Here's the drawing with two shaded views (mm, measured from the low corner). I have some questions. Coordinates: 2 decimals unless noted, no trailing zeros. Loops run counter-clockwise (first coordinate to the right, second up) from the corner with the lowest first, then second, coordinate; pieces in that order, holes last.
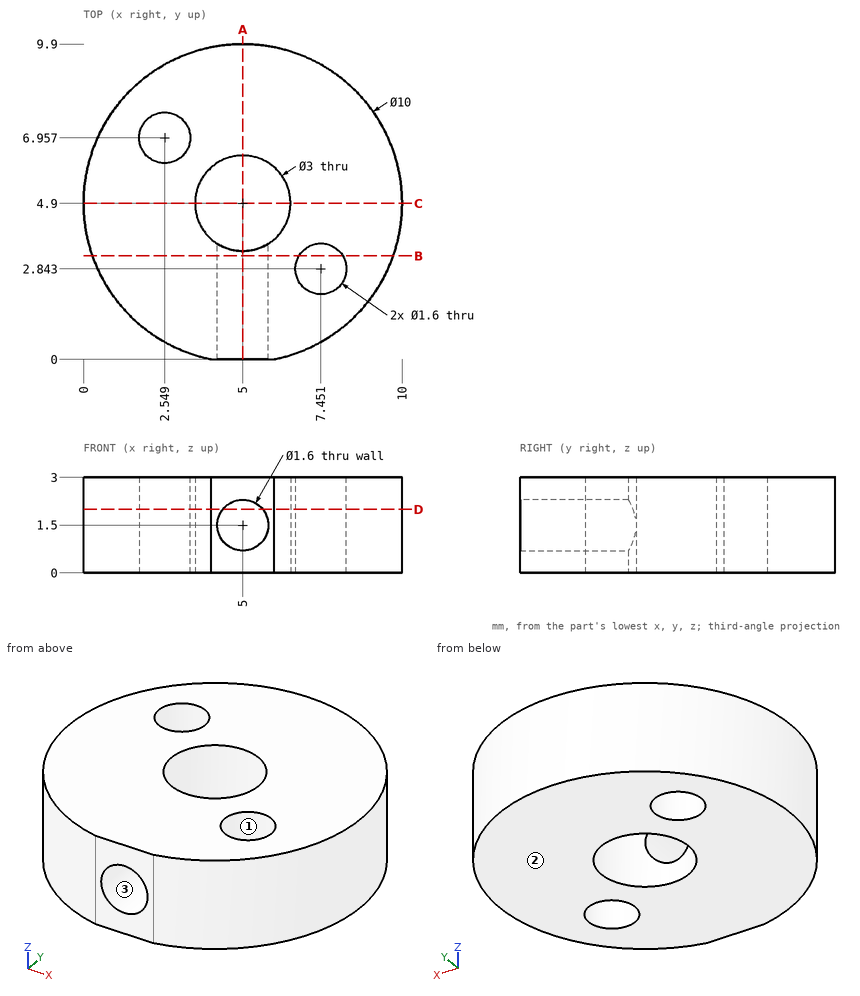
Q1. Suppose I cut it at D-D on z = 2. State how many separate pieces and enclosed holes the cut face has.
Q2. We'd pull the mould along Z, two halves only. Please class the marked faces 1, 2 and 3: pulls with the +Z half, pulls with the -Z half, needs draft (parallel to the pull), parting line crosses it, or undercut.
Q3. Suppose I cut it at A-A on x = 5. Write out the boundary of the cut face in (y, z).
Q4. Suppose I cut it at C-C on y = 4.9. Write out the boundary of the cut face in (x, z).
Q5. Will these pins go through, and if not, where does the flat tip stop? P1, Ø1.5, axis at x = 3.5, z = 1, coming from the +Y side; P2, Ø1.3, axis at x = 7.45, y = 2.84, coming from the +Z side.
Q6. Please list where these lines run through material, in increasing order: probe 1 along X at (y, z) = (1.35, 1.5); probe 2 along X at (y, z) = (1.8, 1.5); probe 3 along Y at (x, z) = (7.5, 2.2) (1 decimal).
Q7. Suppose I cut it at B-B on y = 3.25. Write out the boundary of the cut face in (x, z), and give its area (3 significant figures).
Check values:
1. separate pieces: 1
1. enclosed holes: 2
2. face 1: needs draft
2. face 2: pulls with the -Z half
2. face 3: undercut
3. outline: (0, 0) - (3.4, 0) - (3.4, 0.7) - (0, 0.7) - close; (0, 2.3) - (3.4, 2.3) - (3.4, 3) - (0, 3) - close; (6.4, 0) - (9.9, 0) - (9.9, 3) - (6.4, 3) - close
4. outline: (0, 0) - (3.5, 0) - (3.5, 3) - (0, 3) - close; (6.5, 0) - (10, 0) - (10, 3) - (6.5, 3) - close
5. P1: stops at y = 9.84
5. P2: passes through
6. probe 1: x = 1.48 to 4.2, 5.8 to 8.52
6. probe 2: x = 1.08 to 4.2, 5.8 to 8.92
6. probe 3: y = 0.6 to 2, 3.6 to 9.2
7. outline: (0.28, 0) - (6.76, 0) - (6.76, 3) - (0.28, 3) - close; (8.14, 0) - (9.72, 0) - (9.72, 3) - (8.14, 3) - close; hole circle Ø1.6 at (5, 1.5)
7. area: 22.2 mm2
